```python
from build123d import *

# Parameters (mm, degrees)
F0_R     = 8.980256
F1_DEPTH = 15.875
F2_R     = 3.175
F2_R_2   = 2.38125
F3_DEPTH = 3.175
F4_R     = 2.38125
F5_DEPTH = 1.5875
F7_DEPTH = 12.7


with BuildPart() as f1:
    # F0 (on Top) → F1 (new body)
    with BuildSketch(Plane.XY):
        Circle(F0_R)
    extrude(amount=F1_DEPTH)

    # F2 (on face) → F3 (join)
    with BuildSketch(Plane(origin=(0, 0, 0), x_dir=(1, 0, 0), z_dir=(0, 0, -1))):
        Circle(F2_R)
        Circle(F2_R_2, mode=Mode.SUBTRACT)
    extrude(amount=F3_DEPTH)

    # F4 (on face) → F5 (join)
    with BuildSketch(Plane.XY.offset(15.875)):
        with Locations((-3.96875, 3.96875)):
            Circle(F4_R)
        with Locations((3.96875, 3.96875)):
            Circle(F4_R)
        with Locations((3.96875, -3.96875)):
            Circle(F4_R)
        with Locations((-3.96875, -3.96875)):
            Circle(F4_R)
    extrude(amount=F5_DEPTH)

    # F6 (on Front) → F7 (cut, symmetric)
    with BuildSketch(Plane.XZ):
        with BuildLine():
            ThreePointArc((0, 10.31875), (1.683798, 11.016202), (2.38125, 12.7))
            ThreePointArc((2.38125, 12.7), (-1.683798, 14.383798), (0, 10.31875))
        make_face()
    extrude(amount=F7_DEPTH, both=True, mode=Mode.SUBTRACT)


solid = f1.part
```
Could you check a few things on this model? Use its own coordinates, in mm. A direction names the side the tool comes from. Coordinates: 2 decimals unless noted, no trailing zeros. Write each loop counter-clockwise with the first axis right and the second up, starting at its lowest first coordinate (ties: lowest second). Pieces come first, ordered by that corner, then holes. Notation, with made-up numbers: (79.25, 64.5) -> (125.25, 64.5) arc R16 ccw to (125.25, 71.5) -> close; hole circle Ø11 at (64.25, 79). An arc over 180 degrees is marked (long way). Return JSON: item names as keys, results as strings.
(1) Imagine slicing it at C-C, the plane x = 2.75. Please give me the cut outline in (y, z) (1 decimal), then the cut area to 3 significant figures.
Numbers:
{"outline": "(-8.5, 0) -> (-1.6, 0) -> (-1.6, -3.2) -> (1.6, -3.2) -> (1.6, 0) -> (8.5, 0) -> (8.5, 15.9) -> (6, 15.9) -> (6, 17.5) -> (1.9, 17.5) -> (1.9, 15.9) -> (-1.9, 15.9) -> (-1.9, 17.5) -> (-6, 17.5) -> (-6, 15.9) -> (-8.5, 15.9) -> close", "area": "294 mm2"}
(2) Imagine slicing it at B-B, the plane z = 5.5. Please give me the cut outline in (x, y), then the cut area to 3 significant figures.
Numbers:
{"outline": "circle Ø17.96 at (0, 0)", "area": "253 mm2"}
(3) I need wall thicknesses on L1, parallel to Y at x = 0, z = -1 (3 decimals); L2, parallel to Z at x = -6.75, y = 1 (3 decimals). Which ranges of each line are inside material? Lowest first, please.
Numbers:
{"L1": "y = -3.175 to -2.381, 2.381 to 3.175", "L2": "z = 0 to 15.875"}
(4) Imagine slicing it at D-D, the plane y = 3.5. Please give me the cut outline in (x, z) (1 decimal), then the cut area to 3 significant figures.
Numbers:
{"outline": "(-8.3, 0) -> (8.3, 0) -> (8.3, 15.9) -> (6.3, 15.9) -> (6.3, 17.5) -> (1.6, 17.5) -> (1.6, 15.9) -> (-1.6, 15.9) -> (-1.6, 17.5) -> (-6.3, 17.5) -> (-6.3, 15.9) -> (-8.3, 15.9) -> close; hole circle Ø4.8 at (0, 12.7)", "area": "260 mm2"}
(5) We'd pull the mould along Y, two halves only. Please class faces 1 (the cylindrical face through (8.566, 2.697, 7.826)), 2 (the flat face through (4, 4, 17.462)), 3 (the cylindrical face through (6.24, -3.25, 16.66)), 4 (the flat face through (0, 0, 0)): +Y half, -Y half, draft (parallel to the pull), parting line (faces both ways), or undercut.
Numbers:
{"face 1": "parting line", "face 2": "draft", "face 3": "undercut", "face 4": "undercut"}
(6) Which directions (+Z, -Z, +X, -X, +Y, -Y) give clear straight access to the entire face, cutting with the end or side of a thin tool? Please do faces 5 (the flat face through (4, 0, 0)), 6 (the flat face through (-4, 4, 17.462)), 7 (the flat face through (0, 0, 15.875)).
Numbers:
{"face 5": "-Z", "face 6": "+Z, +X, -X, +Y, -Y", "face 7": "+Z"}
(7) I'm going to push flat-ended pins straight in: pin 1 (8 mm diameter, centred on y = 3.5, z = 1, fed in from +X); pin 2 (3 mm diameter, centred on y = -5.5, z = 4, fed in from -X); pin 3 (5 mm diameter, centred on y = 5.5, z = 8, fed in from +X); pin 4 (2 mm diameter, centred on x = -3, y = 5, fed in from -Z). Where does each tip first touch, or does it pass through?
Numbers:
{"pin 1": "stops at x = 8.98", "pin 2": "stops at x = -8.04", "pin 3": "stops at x = 8.46", "pin 4": "stops at z = 0"}
(8) Imagine slicing it at A-A, the plane y = 0. Please give me the cut outline in (x, z) (1 decimal).
Numbers:
{"outline": "(-9, 0) -> (-3.2, 0) -> (-3.2, -3.2) -> (-2.4, -3.2) -> (-2.4, 0) -> (2.4, 0) -> (2.4, -3.2) -> (3.2, -3.2) -> (3.2, 0) -> (9, 0) -> (9, 15.9) -> (-9, 15.9) -> close; hole circle Ø4.8 at (0, 12.7)"}
